Verification items for the finished model (mm, model axes). Face numbers are marked on the shaded views. Round coordinates to 2 decimals unless told otherwise and drop trailing zeros. Order: outer loops, then holes, each group sorted by start corner. A loop starts at its lowest first (then second) coordinate and runs counter-clockwise, first axis right, second up. Notation, with made-up numbers: M -7,22 L 49,22 A24 cw 49,44 Z; hole C 75.5,-29.5 d9. An arc over 180 degrees is marked long. One line per item, written item: value. Start each with the question number.
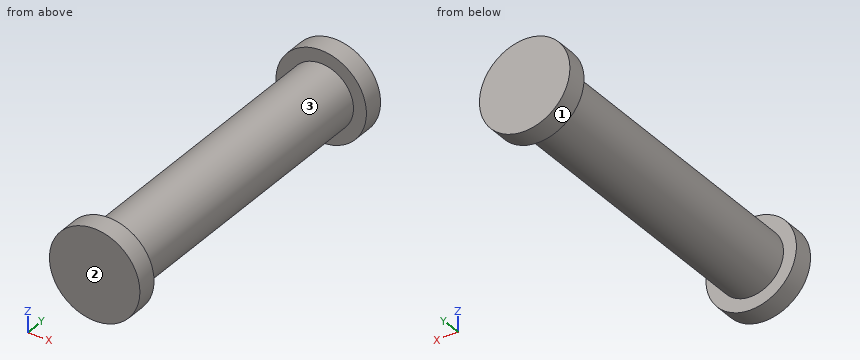
from build123d import *

# Parameters (mm, degrees)
F0_R      = 3.175
F1_DEPTH  = 10
F1_FACE_R = 3.175
F2_R      = 4.445
F3_DEPTH  = 2
F4_DEPTH  = 20
F5_R      = 4.445
F6_DEPTH  = 2


with BuildPart() as f1:
    # F0 (on Front) → F1 (new body)
    with BuildSketch(Plane.XZ):
        with Locations((-68.0588558316, 31.7334979773)):
            Circle(F0_R)
    extrude(amount=F1_DEPTH)

    # F1_face (on face) + F2 (on face) → F3 (join)
    with BuildSketch(Plane(origin=(-68.0588558316, -10, 31.7334979773), x_dir=(1, 0, 0), z_dir=(0, -1, 0))):
        Circle(F1_FACE_R)
    with BuildSketch(Plane.XZ.offset(10)):
        with Locations((-68.0588558316, 31.7334979773)):
            Circle(F2_R)
    extrude(amount=F3_DEPTH)

    # F4 (add): a face of the model
    f4_faces = [f1.faces().sort_by_distance(p)[0] for p in [
        (-68.0588558316, 0, 31.7334979773),
    ]]
    extrude(f4_faces, amount=F4_DEPTH)

    # F5 (on face) → F6 (join)
    with BuildSketch(Plane(origin=(0, 20, 0), x_dir=(-1, 0, 0), z_dir=(0, 1, 0))):
        with Locations((68.0588558316, 31.7334979773)):
            Circle(F5_R)
    extrude(amount=F6_DEPTH)


solid = f1.part
1. Section check B-B (z = 33.5). Record the cut outline in (x, y).
2. Scan lines: line 1 along Y through (x, z) = (-71.25, 34); line 2 along Z through (x, y) = (-68, -1.5); line 3 along Z through (x, y) = (-66.5, 19.5). Record each from-to range of solid material in increasing order.
3. Depth check by flat-ended pin: pin 1 (3 mm diameter, centred on y = 17, z = 32, fed in from -X); pin 2 (1.5 mm diameter, centred on y = 9, z = 34, fed in from +X); pin 3 (1.5 mm diameter, centred on y = 10.5, z = 30, fed in from +X). Enter the tip coordinate at first touch or a pass-through.
4. Section check A-A (x = -67). Record the cut outline in (y, z), and give its area (3 significant figures).
5. Draft check along Y on the marked faces 1, 2 and 3. Enter one of: released by +Y, released by -Y, zero draft, split by the parting line, or undercut.
Geometry check:
1. outline: M -72.14,-12 L -63.98,-12 L -63.98,-10 L -65.42,-10 L -65.42,20 L -63.98,20 L -63.98,22 L -72.14,22 L -72.14,20 L -70.7,20 L -70.7,-10 L -72.14,-10 Z
2. line 1: y = -12 to -10, 20 to 22
2. line 2: z = 28.56 to 34.91
2. line 3: z = 28.97 to 34.5
3. pin 1: stops at x = -71.23
3. pin 2: stops at x = -65.27
3. pin 3: stops at x = -65.04
4. outline: M -12,27.42 L -10,27.42 L -10,28.74 L 20,28.74 L 20,27.42 L 22,27.42 L 22,36.05 L 20,36.05 L 20,34.73 L -10,34.73 L -10,36.05 L -12,36.05 Z
4. area: 214 mm²
5. face 1: zero draft
5. face 2: released by -Y
5. face 3: undercut
